Check sheet for the modelled part. Datum: model origin and axes. Units: mm. A direction names the side the tool comes from. Coordinates: 2 decimals unless noted, no trailing zeros. Loops run counter-clockwise (first coordinate to the right, second up) from the corner with the lowest first, then second, coordinate; pieces in that order, holes last. Notation, with made-up numbers: (56.25, -9.75) -> (93.25, -9.75) arc R28 cw to (93.25, 26.25) -> close; hole circle Ø3 at (84.5, 62.25). An arc over 180 degrees is marked (long way). Use CSV: the item, a comma, the result in double quotes. Start each with the question number.
1. Sectioned sample at D-D, the plane z = 197. Record the cut outline in (x, y), and give its area (3 significant figures).
2. Sectioned sample at C-C, the plane x = -20.5. Record the cut outline in (y, z).
3. Gauge pin test, flat ends, axial feed: pin 1 (3 mm diameter, centred on x = -162, z = 199.5, fed in from -Y); pin 2 (5 mm diameter, centred on y = 17, z = 170.5, fed in from -X); pin 3 (1.5 mm diameter, centred on x = 110, y = 50.5, fed in from -Z); pin 4 (5 mm diameter, centred on x = 237, z = -54, fed in from -Y). Record the tip position at first contact, or that the pin passes through.
4. Release check for a two-part mould opening along Y. For faces 6 (the face through (78.1, 13.28, 17.34)), 7 (the face through (197, 46.2, -1)), 8 (the face through (119.74, 87.68, -234.07)) record: pulls with the +Y half, pulls with the -Y half, needs draft (parallel to the pull), parting line crosses it, or undercut.
5. Sectioned sample at B-B, the plane y = 9. Record the cut outline in (x, z), and give its area (3 significant figures).
6. Sectioned sample at A-A, the plane x = 183. Record the cut outline in (y, z).
7. Set-up check for faces 1 (the face through (101, 78, -249)), 2 (the face through (-200, 39, 42)), 3 (the face through (-71.5, 36.2, -23.3)), 4 (the face through (74.5, 55, -229)), 5 (the face through (114, 96, -229)): record each of +Z, -Z, +X, -X, +Y, -Y from which the full face is reachable in a straight line by a thin tool's end or side.
8. Thickness scan on L1, parallel to X at y = 33.8, z = 0; L2, parallel to X at y = 9, z = 0; L3, parallel to X at y = 47, z = -54. Record the ranges inside material, lowest first.
```python
from build123d import *

# Parameters (mm, degrees)
SKETCH_1_R          = 305
EXTRUDE_1_DEPTH     = 41.2
SKETCH_2_W          = 140
SKETCH_2_H          = 140
EXTRUDE_2_DEPTH     = 10
SHELL_1_T           = -5
CUT_EXTRUDE_1_DEPTH = 434.298326791
SKETCH_4_W          = 120
SKETCH_4_H          = 10
EXTRUDE_3_DEPTH     = 150
CUT_EXTRUDE_3_DEPTH = 150
SKETCH_6_R          = 10
CUT_EXTRUDE_4_DEPTH = 150
SKETCH_7_R          = 20
SKETCH_7_R_2        = 10
EXTRUDE_4_DEPTH     = 10
SKETCH_8_W          = 5
SKETCH_8_H          = 36
SKETCH_8_W_2        = 7.838760884
EXTRUDE_5_DEPTH     = 26
CUT_EXTRUDE_5_DEPTH = 535.481627176
SKETCH_11_W         = 19
SKETCH_11_H         = 5
SKETCH_11_W_2       = 5
SKETCH_11_H_2       = 46.5
SKETCH_18_R         = 4
SKETCH_18_R_2       = 8
CUT_EXTRUDE_9_DEPTH = 440.824965185


with BuildPart() as part:
    # 草图1 → 凸台-拉伸1 (new body)
    with BuildSketch(Plane(origin=(0, 0, 0), x_dir=(1, 0, 0), z_dir=(0, 1, 0))):
        with Locations(Location((0, 0, 0), (0, 0, 90))):
            Circle(SKETCH_1_R)
    extrude(amount=EXTRUDE_1_DEPTH)

    # 草图2 → 凸台-拉伸2 (add)
    with BuildSketch(Plane(origin=(0, 41.2, 0), x_dir=(1, 0, 0), z_dir=(0, 1, 0))):
        with Locations((183, 0)):
            Rectangle(SKETCH_2_W, SKETCH_2_H)
    extrude(amount=EXTRUDE_2_DEPTH)

    # 抽壳1
    shell_1_openings = [part.faces().sort_by_distance(p)[0] for p in [
        (0, 0, 0),
    ]]
    offset(amount=SHELL_1_T, openings=shell_1_openings, kind=Kind.INTERSECTION)

    # 草图3 → 切除-拉伸1 (cut, through all)
    with BuildSketch(Plane(origin=(0, 41.2, 0), x_dir=(1, 0, 0), z_dir=(0, 1, 0))):
        with BuildLine():
            Line((-182, -24), (-118, -24))
            ThreePointArc((-118, -24), (-100, -42), (-118, -60))
            Line((-118, -60), (-182, -60))
            ThreePointArc((-182, -60), (-200, -42), (-182, -24))
        make_face()
    extrude(amount=-CUT_EXTRUDE_1_DEPTH, mode=Mode.SUBTRACT)

    # 草图4 → 凸台-拉伸3 (add)
    with BuildSketch(Plane(origin=(0, 41.2, 0), x_dir=(1, 0, 0), z_dir=(0, 1, 0))):
        with Locations((99, 244)):
            Rectangle(SKETCH_4_W, SKETCH_4_H)
    extrude(amount=EXTRUDE_3_DEPTH)

    # 草图5 → 切除-拉伸3 (cut)
    with BuildSketch(Plane.XY.offset(-239)):
        with BuildLine():
            Line((39, 191.2), (39, 41.2))
            ThreePointArc((39, 41.2), (53.931588882, 82.177347592), (74.646786984, 120.556716136))
            ThreePointArc((74.646786984, 120.556716136), (115.26317996, 135.706044936), (140.99801314, 100.821780537))
            ThreePointArc((140.99801314, 100.821780537), (138.32356193, 70.621084147), (131, 41.2))
            Line((131, 41.2), (159, 41.2))
            Line((159, 41.2), (159, 191.2))
            Line((159, 191.2), (39, 191.2))
        make_face()
    extrude(amount=-CUT_EXTRUDE_3_DEPTH, mode=Mode.SUBTRACT)

    # 草图6 → 切除-拉伸4 (cut)
    with BuildSketch(Plane.XY.offset(-239)):
        with Locations((105, 101.2)):
            Circle(SKETCH_6_R)
    extrude(amount=-CUT_EXTRUDE_4_DEPTH, mode=Mode.SUBTRACT)

    # 草图7 → 凸台-拉伸4 (add)
    with BuildSketch(Plane.XY.offset(-239)):
        with Locations(Location((105, 101.2, 0), (0, 0, 180))):
            Circle(SKETCH_7_R)
        with Locations((105, 101.2)):
            Circle(SKETCH_7_R_2, mode=Mode.SUBTRACT)
    extrude(amount=EXTRUDE_4_DEPTH)

    # 草图8 → 凸台-拉伸5 (add)
    with BuildSketch(Plane.XY.offset(-239)):
        with Locations((72, 59.2)):
            Rectangle(SKETCH_8_W, SKETCH_8_H)
        with Locations((108, 59.2)):
            Rectangle(SKETCH_8_W_2, SKETCH_8_H)
    extrude(amount=EXTRUDE_5_DEPTH)

    # 草图10 → 切除-拉伸5 (cut, through all)
    with BuildSketch(Plane(origin=(111.919380442, 0, 0), x_dir=(0, 0, -1), z_dir=(1, 0, 0))):
        Polygon((213, 41.2), (239, 77.2), (213, 77.2), align=None)
    extrude(amount=-CUT_EXTRUDE_5_DEPTH, mode=Mode.SUBTRACT)

    # 草图11 → 旋转1 (revolve)
    with BuildSketch(Plane.XY, mode=Mode.PRIVATE) as revolve_1_sk:
        with Locations((-65.5, 33.7)):
            Rectangle(SKETCH_11_W, SKETCH_11_H)
        with Locations((-82.5, 12.95)):
            Rectangle(SKETCH_11_W_2, SKETCH_11_H_2)
    revolve(revolve_1_sk.sketch.rotate(Axis((0, 0, 0), (0, 1, 0)), 270), axis=Axis((0, 0, 0), (0, 1, 0)))

    # 草图18 → 切除-拉伸9 (cut, through all)
    with BuildSketch(Plane(origin=(0, 51.2, 0), x_dir=(1, 0, 0), z_dir=(0, 1, 0))):
        with Locations(Location((237, 54, 0), (0, 0, 270))):
            Circle(SKETCH_18_R)
        with Locations(Location((237, -54, 0), (0, 0, 270))):
            Circle(SKETCH_18_R)
        with Locations(Location((129, -54, 0), (0, 0, 270))):
            Circle(SKETCH_18_R)
        with Locations(Location((129, 54, 0), (0, 0, 270))):
            Circle(SKETCH_18_R)
        with Locations(Location((183, 0, 0), (0, 0, 270))):
            Circle(SKETCH_18_R_2)
    extrude(amount=-CUT_EXTRUDE_9_DEPTH, mode=Mode.SUBTRACT)


solid = part.part
```
Completed:
1,outline,"(-232.84, 0) -> (-226.25, 0) -> (-226.25, 36.2) -> (226.25, 36.2) -> (226.25, 0) -> (232.84, 0) -> (232.84, 41.2) -> (-232.84, 41.2) -> close"
1,area,"2,810 mm²"
2,outline,"(-10.3, -82.49) -> (36.2, -82.49) -> (36.2, -299.3) -> (0, -299.3) -> (0, -304.31) -> (41.2, -304.31) -> (41.2, 304.31) -> (0, 304.31) -> (0, 299.3) -> (36.2, 299.3) -> (36.2, 82.49) -> (-10.3, 82.49) -> (-10.3, 77.33) -> (36.2, 77.33) -> (36.2, 72.14) -> (31.2, 72.14) -> (31.2, 52.11) -> (36.2, 52.11) -> (36.2, -52.11) -> (31.2, -52.11) -> (31.2, -72.14) -> (36.2, -72.14) -> (36.2, -77.33) -> (-10.3, -77.33) -> close"
3,pin 1,"y = 36.2"
3,pin 2,"x = -254.56"
3,pin 3,"z = -249"
3,pin 4,"through"
4,face 6,"needs draft"
4,face 7,"pulls with the -Y half"
4,face 8,"undercut"
5,outline,"circle Ø610 at (0, 0); circle Ø170 at (0, 0); hole circle Ø600 at (0, 0); hole circle Ø160 at (0, 0)"
5,area,"12,100 mm²"
6,outline,"(0, -244) -> (41.2, -244) -> (41.2, -70) -> (51.2, -70) -> (51.2, -8) -> (46.2, -8) -> (46.2, -65) -> (36.2, -65) -> (36.2, -237.72) -> (0, -237.72) -> close; (0, 237.72) -> (36.2, 237.72) -> (36.2, 65) -> (46.2, 65) -> (46.2, 8) -> (51.2, 8) -> (51.2, 70) -> (41.2, 70) -> (41.2, 244) -> (0, 244) -> close"
7,face 1,"-Z, +X, -X, +Y"
7,face 2,"+Y, -Y"
7,face 3,"-Y"
7,face 4,"+Z, +Y"
7,face 5,"+Z, +X, -X, +Y"
8,L1,"-305 to -300, -85 to -80, -75 to -56, 56 to 75, 80 to 85, 300 to 305"
8,L2,"-305 to -300, -85 to -80, 80 to 85, 300 to 305"
8,L3,"113 to 125, 133 to 233, 241 to 253"
